The listing builds one solid part. Answer for the finished solid, in the listing's coordinates (mm). A direction names the side the tool comes from. Give positions to 0.01 mm unless a question says otherwise; leave off trailing zeros. Use a Markdown table: item, result. Add a question column.
1) For faces 1 (the face through (126.302, 7.745, -35.855)), 2 (the face through (146.502, 4.408, -41.512)), 3 (the face through (107.42, -0.77, -109.19)), determine the directions among +Z, -Z, +X, -X, +Y, -Y from which every point of the face is accessible in a straight line to the end or side of a thin tool.
2) Straight lines are drawn through the part: line 1 (Z direction, x = 152, y = 7); line 2 (X direction, y = 14.75, z = -132); line 3 (Y direction, x = 102, z = -96). For each, find the intervals that lie inside material, in ascending order.
3) Flat-ended cylindrical pins translate along their axes: pin 1 (1.5 mm diameter, centred on y = 14.5, z = -120, fed in from -X); pin 2 (3 mm diameter, centred on x = 141.5, z = -46, fed in from +Y); pin 3 (3 mm diameter, centred on x = 99.5, z = -127, fed in from -Y). Find the tip coordinate at first contact, or state that the pin passes through.
4) The mould has two halves that part along Z. Classify faces 4 (the face through (106.844, 5.434, -82.009)), 5 (the face through (130.21, 7.72, -29.22)), 6 (the face through (110.76, 5.51, -109.15)): released by +Z, released by -Z, zero draft, split by the parting line, or undercut.
from build123d import *

# Parameters (mm, degrees)
BOSS_EXTRUDE1_DEPTH      = 4
BOSS_EXTRUDE2_DEPTH      = 14
CUT_EXTRUDE3_DEPTH       = 15
CUT_EXTRUDE4_DEPTH       = 5
SKETCH7_R                = 2.125
CUT_EXTRUDE5_DEPTH       = 4
SKETCH8_R                = 2.125
CUT_EXTRUDE6_DEPTH       = 4
FILLET1_R                = 3
CHAMFER1_SIZE            = 1.5
BOSS_EXTRUDE3_DEPTH      = 40.85
BOSS_EXTRUDE3_DEPTH_BACK = 40.85
CUT_EXTRUDE7_DEPTH       = 76.384173958
CUT_EXTRUDE7_DEPTH_BACK  = 81.869001515
CUT_EXTRUDE8_DEPTH       = 3.3077
BOSS_EXTRUDE4_DEPTH      = 4
BOSS_EXTRUDE5_DEPTH      = 81.7
CUT_EXTRUDE9_DEPTH       = 30.834988393
SKETCH16_R               = 1.25
BOSS_EXTRUDE6_DEPTH      = 4
CUT_EXTRUDE10_DEPTH      = 35.534173958
CUT_EXTRUDE10_DEPTH_BACK = 122.719001515


with BuildPart() as part:
    # Sketch1 → Boss-Extrude1 (new body)
    with BuildSketch(Plane(origin=(0, 0, 0), x_dir=(1, 0, 0), z_dir=(0, 1, 0))):
        Polygon((81.735026919, 121.569219382), (146.149545762, 10), (170.398257068, 10), (93.859382572, 142.569219382), align=None)
    extrude(amount=BOSS_EXTRUDE1_DEPTH)

    # Sketch2 → Boss-Extrude2 (add)
    with BuildSketch(Plane(origin=(0, 4, 0), x_dir=(1, 0, 0), z_dir=(0, 1, 0))):
        Polygon((93.859382572, 142.569219382), (81.735026919, 121.569219382), (84.044427996, 117.569219382), (96.168783649, 138.569219382), align=None)
        Polygon((146.149545762, 10), (170.398257068, 10), (168.088855991, 14), (143.840144685, 14), align=None)
    extrude(amount=BOSS_EXTRUDE2_DEPTH)

    # Sketch5 → Cut-Extrude3 (cut, through all)
    with BuildSketch(Plane(origin=(0, 4, 0), x_dir=(1, 0, 0), z_dir=(0, 1, 0))):
        Polygon((96.168783649, 138.569219382), (92.704682034, 140.569219382), (93.859382572, 142.569219382), align=None)
        Polygon((81.735026919, 121.569219382), (85.199128534, 119.569219382), (84.044427996, 117.569219382), align=None)
        Polygon((146.149545762, 10), (146.149545762, 14), (143.840144685, 14), align=None)
        Polygon((168.088855991, 14), (168.088855991, 10), (170.398257068, 10), align=None)
    extrude(amount=CUT_EXTRUDE3_DEPTH, mode=Mode.SUBTRACT)

    # Sketch6 → Cut-Extrude4 (cut, through all)
    with BuildSketch(Plane(origin=(0, 4, 0), x_dir=(1, 0, 0), z_dir=(0, 1, 0))):
        Polygon((93.859382572, 142.569219382), (96.168783649, 138.569219382), (92.704682034, 140.569219382), align=None)
        Polygon((168.088855991, 14), (168.088855991, 10), (170.398257068, 10), align=None)
    extrude(amount=-CUT_EXTRUDE4_DEPTH, mode=Mode.SUBTRACT)

    # Sketch7 → Cut-Extrude5 (cut)
    with BuildSketch(Plane.XY.offset(-10)):
        with Locations((157.119200877, 10)):
            Circle(SKETCH7_R)
    extrude(amount=-CUT_EXTRUDE5_DEPTH, mode=Mode.SUBTRACT)

    # Sketch8 → Cut-Extrude6 (cut)
    with BuildSketch(Plane(origin=(8.660254038, 0, 5), x_dir=(-0.5, 0, 0.866025404), z_dir=(-0.866025404, 0, -0.5))):
        with Locations((-157.119200877, 10)):
            Circle(SKETCH8_R)
    extrude(amount=-CUT_EXTRUDE6_DEPTH, mode=Mode.SUBTRACT)

    # Fillet1
    fillet1_edges = [part.edges().sort_by_distance(p)[0] for p in [
        (94.436732841, 18, -139.569219382),
        (83.467077727, 18, -120.569219382),
        (146.149545762, 18, -12),
        (168.088855991, 18, -12),
    ]]
    fillet(fillet1_edges, radius=FILLET1_R)

    # Chamfer1
    chamfer1_edges = [part.edges().sort_by_distance(p)[0] for p in [
        (96.168783649, 9.5, -138.569219382),
        (85.199128534, 9.5, -119.569219382),
        (90.683956091, 18, -129.069219382),
        (85.638468362, 17.121320344, -120.330178286),
        (95.72944382, 17.121320344, -137.808260477),
        (146.149545762, 9.5, -14),
        (157.119200877, 18, -14),
        (168.088855991, 9.5, -14),
        (167.210176335, 17.121320344, -14),
        (147.028225419, 17.121320344, -14),
    ]]
    chamfer(chamfer1_edges, length=CHAMFER1_SIZE)

    # Sketch10 → Boss-Extrude3 (add, two sides)
    with BuildSketch(Plane(origin=(0, 0, 0), x_dir=(0.866025404, 0, -0.5), z_dir=(0.5, 0, 0.866025404))) as boss_extrude3_sk:
        Polygon((152.569219382, 4), (131.569219382, 4), (129.026250632, 4.943910052), (131.569219382, 11.794870108), align=None)
    extrude(amount=BOSS_EXTRUDE3_DEPTH)
    extrude(boss_extrude3_sk.sketch, amount=-BOSS_EXTRUDE3_DEPTH_BACK)

    # Sketch11 → Cut-Extrude7 (cut, two sides)
    with BuildSketch(Plane(origin=(0, 0, 0), x_dir=(0.866025404, 0, -0.5), z_dir=(0.5, 0, 0.866025404))) as cut_extrude7_sk:
        Polygon((152.569219382, 4), (151.084482218, 0), (152.569219382, 0), align=None)
    extrude(amount=CUT_EXTRUDE7_DEPTH, mode=Mode.SUBTRACT)
    extrude(cut_extrude7_sk.sketch, amount=-CUT_EXTRUDE7_DEPTH_BACK, mode=Mode.SUBTRACT)

    # Sketch12 → Cut-Extrude8 (cut)
    with BuildSketch(Plane(origin=(17.130089599, 53.289226321, -9.890061841), x_dir=(0.953509144, -0.29630427, 0.054991745), z_dir=(0.301364086, 0.9375, -0.173992636))):
        Polygon((80.111656223, 97.310988855), (99.184922165, 109.057074429), (142.026671782, 39.490742847), (122.95340584, 27.744657273), align=None)
    extrude(amount=-CUT_EXTRUDE8_DEPTH, mode=Mode.SUBTRACT)

    # Sketch14 → Boss-Extrude4 (add)
    with BuildSketch(Plane(origin=(16.13326761, 50.188257571, -9.314546398), x_dir=(0.953509144, -0.29630427, 0.054991745), z_dir=(0.301364086, 0.9375, -0.173992636))):
        with BuildLine():
            Line((80.111656223, 97.310988855), (84.539378674, 100.037758721))
            Line((84.539378674, 100.037758721), (85.850325725, 97.909046004))
            ThreePointArc((85.850325725, 97.909046004), (86.032422143, 96.775529185), (85.359666325, 95.845250143))
            Line((85.359666325, 95.845250143), (82.209171505, 93.905048508))
            Line((82.209171505, 93.905048508), (80.111656223, 97.310988855))
        make_face()
        with BuildLine():
            Line((99.184922165, 109.057074429), (94.757199714, 106.330304564))
            Line((94.757199714, 106.330304564), (96.068146765, 104.201591847))
            ThreePointArc((96.068146765, 104.201591847), (96.998425806, 103.52883603), (98.131942626, 103.710932448))
            Line((98.131942626, 103.710932448), (101.282437446, 105.651134083))
            Line((101.282437446, 105.651134083), (99.184922165, 109.057074429))
        make_face()
        with BuildLine():
            Line((122.95340584, 27.744657273), (120.855890559, 31.15059762))
            Line((120.855890559, 31.15059762), (124.00638538, 33.090799255))
            ThreePointArc((124.00638538, 33.090799255), (125.139902199, 33.272895673), (126.07018124, 32.600139855))
            Line((126.07018124, 32.600139855), (127.381128291, 30.471427139))
            Line((127.381128291, 30.471427139), (122.95340584, 27.744657273))
        make_face()
        with BuildLine():
            Line((142.026671782, 39.490742847), (137.598949331, 36.763972982))
            Line((137.598949331, 36.763972982), (136.28800228, 38.892685699))
            ThreePointArc((136.28800228, 38.892685699), (136.105905862, 40.026202518), (136.77866168, 40.956481559))
            Line((136.77866168, 40.956481559), (139.929156501, 42.896683194))
            Line((139.929156501, 42.896683194), (142.026671782, 39.490742847))
        make_face()
    extrude(amount=BOSS_EXTRUDE4_DEPTH)

    # Sketch15 → Boss-Extrude5 (add)
    with BuildSketch(Plane(origin=(20.425, 0, 35.377137745), x_dir=(0.866025404, 0, -0.5), z_dir=(0.5, 0, 0.866025404))):
        Polygon((129.026250632, 4.943910052), (150.026250632, -2.850960056), (151.084482218, 0), align=None)
    extrude(amount=-BOSS_EXTRUDE5_DEPTH)

    # Sketch13 → Cut-Extrude9 (cut, through all)
    with BuildSketch(Plane(origin=(16.13326761, 50.188257571, -9.314546398), x_dir=(0.953509144, -0.29630427, 0.054991745), z_dir=(0.301364086, 0.9375, -0.173992636))):
        with BuildLine():
            Line((94.663168486, 73.6822777), (101.47504918, 77.877308262))
            ThreePointArc((101.47504918, 77.877308262), (102.211038279, 80.973002053), (99.115344488, 81.708991152))
            Line((99.115344488, 81.708991152), (92.303463795, 77.51396059))
            Line((92.303463795, 77.51396059), (94.663168486, 73.6822777))
        make_face()
    extrude(amount=-CUT_EXTRUDE9_DEPTH, mode=Mode.SUBTRACT)

    # Sketch16 → Boss-Extrude6 (add)
    with BuildSketch(Plane(origin=(16.13326761, 50.188257571, -9.314546398), x_dir=(0.953509144, -0.29630427, 0.054991745), z_dir=(0.301364086, 0.9375, -0.173992636))):
        with BuildLine():
            Line((99.735519926, 108.163015088), (104.078093869, 110.837347072))
            ThreePointArc((104.078093869, 110.837347072), (109.37516991, 109.577987946), (108.115810785, 104.280911904))
            Line((108.115810785, 104.280911904), (103.773236843, 101.606579921))
            Line((103.773236843, 101.606579921), (99.735519926, 108.163015088))
        make_face()
        with Locations((106.096952327, 107.559129488)):
            Circle(SKETCH16_R, mode=Mode.SUBTRACT)
        with BuildLine():
            Line((76.319680043, 93.742597531), (80.662253985, 96.416929514))
            Line((80.662253985, 96.416929514), (84.699970901, 89.860494347))
            Line((84.699970901, 89.860494347), (80.357396959, 87.186162363))
            ThreePointArc((80.357396959, 87.186162363), (75.060320917, 88.445521489), (76.319680043, 93.742597531))
        make_face()
        with Locations((78.338538501, 90.464379947)):
            Circle(SKETCH16_R, mode=Mode.SUBTRACT)
        with BuildLine():
            Line((141.47607402, 40.384802188), (145.818647962, 43.059134172))
            ThreePointArc((145.818647962, 43.059134172), (147.078007088, 48.356210213), (141.780931046, 49.615569339))
            Line((141.780931046, 49.615569339), (137.438357104, 46.941237356))
            Line((137.438357104, 46.941237356), (141.47607402, 40.384802188))
        make_face()
        with Locations((143.799789504, 46.337351755)):
            Circle(SKETCH16_R, mode=Mode.SUBTRACT)
        with BuildLine():
            Line((118.365091163, 35.195151782), (122.402808079, 28.638716614))
            Line((122.402808079, 28.638716614), (118.060234137, 25.964384631))
            ThreePointArc((118.060234137, 25.964384631), (112.763158095, 27.223743756), (114.02251722, 32.520819798))
            Line((114.02251722, 32.520819798), (118.365091163, 35.195151782))
        make_face()
        with Locations((116.041375678, 29.242602214)):
            Circle(SKETCH16_R, mode=Mode.SUBTRACT)
    extrude(amount=-BOSS_EXTRUDE6_DEPTH)

    # Sketch18 → Cut-Extrude10 (cut, two sides)
    with BuildSketch(Plane(origin=(20.425, 0, 35.377137745), x_dir=(0.866025404, 0, -0.5), z_dir=(0.5, 0, 0.866025404))) as cut_extrude10_sk:
        Polygon((131.569219382, 4), (142.345537503, 0), (131.569219382, 0), align=None)
    extrude(amount=CUT_EXTRUDE10_DEPTH, mode=Mode.SUBTRACT)
    extrude(cut_extrude10_sk.sketch, amount=-CUT_EXTRUDE10_DEPTH_BACK, mode=Mode.SUBTRACT)


solid = part.part
The answers:
| question | item | result |
|---|---|---|
| 1 | face 1 | -X, +Y |
| 1 | face 2 | +Y |
| 1 | face 3 | -Z, -X, -Y |
| 2 | line 1 | -14 to -10 |
| 2 | line 2 | 87.76 to 92.38 |
| 2 | line 3 | 2.23 to 6.5 |
| 3 | pin 1 | x = 83.15 |
| 3 | pin 2 | y = 3.64 |
| 3 | pin 3 | y = 0 |
| 4 | face 4 | undercut |
| 4 | face 5 | released by +Z |
| 4 | face 6 | released by -Z |
